Input: part model. Units: mm. Frame: model coordinates. A direction names the side the tool comes from. Coordinates: 2 decimals unless noted, no trailing zeros. Use one line per item in the form item = value.
Autodesk Inventor part; units mm, degrees
ref_plane "YZ Plane" through (0, 0, 0) normal (1, 0, 0) x (0, 1, 0)
ref_plane "XZ Plane" through (0, 0, 0) normal (0, 1, 0) x (-1, 0, 0)
ref_plane "XY Plane" through (0, 0, 0) normal (0, 0, 1) x (1, 0, 0)
ref_plane "Work Plane1" through (-701.2547, 0, 0) normal (0, 0, 1) x (1, 0, 0)
sketch "Sketch1" plane through (-701.2547, 0, 0) normal (0, 0, 1) x (1, 0, 0)
  line L0 (557.3903, 26) -> (429.8698, 26)
  arc A0 (429.8698, 26) -> (429.8698, 4) centre (429.8698, 15) ccw
  line L1 (429.8698, 4) -> (557.3903, 4)
  arc A1 (557.3903, 4) -> (557.3903, 26) centre (557.3903, 15) ccw
  line L2 (701.2547, 0) -> (1.2547, 0)
  line L3 (1.2547, 0) -> (1.2547, 30)
  line L4 (1.2547, 30) -> (701.2547, 30)
  line L5 (701.2547, 30) -> (701.2547, 0)
  line L6 (1.2547, 0) -> (701.2547, 0)
  line L7 (701.2547, 0) -> (701.2547, -50)
  line L8 (701.2547, -50) -> (1.2547, -50)
  line L9 (1.2547, -50) -> (1.2547, 0)
  line L10 (1.2547, -50) -> (31.2547, -700) construction
  line L11 (31.2547, -700) -> (351.2547, -850) construction
  line L12 (351.2547, -850) -> (671.2547, -700) construction
  line L13 (671.2547, -700) -> (701.2547, -50) construction
  spline S0 degree 4 poles (1.2547, -50) (31.2547, -700) (351.2547, -850) (671.2547, -700) (701.2547, -50) knots 1 1 1 1 1 2 2 2 2 2
  dimension "d0" = 50
  dimension "d1" = 850
  dimension "d2" = 700
  dimension "d3" = 30
  dimension "d4" = 30
  dimension "d5" = 350
  dimension "d6" = 350
extrude "Extrusion1" add sketch "Sketch1" along normal blind 25 contours L7 L8 L9 L2 | S0 L8
ref_plane "Work Plane2" through (-700, 0, 1930) normal (-1, 0, 0) x (0, 1, 0)
sketch "Sketch3" plane through (-700, -50, 0) normal (-1, 0, 0) x (0, 0, 1)
  circle A0 centre (37.5, 36) radius 12.5
  line L0 (0, 50) -> (25, 50)
  line L1 (25, 50) -> (25, 0)
  circle A1 centre (37.5, 36) radius 10
  arc A2 (40.5, 23.8653) -> (25, 13.8653) centre (45.3472, -0.6603) ccw
  line L2 (37.5, 48.5) -> (25, 48.5)
  point P0 (12.5, 50)
  point P1 (39.7301, 23.7006)
  point P2 (25, 36)
  point P3 (25, 41.0707)
  dimension "d11" = 12.5
  dimension "d12" = 2.5
  dimension "d13" = 20
  dimension "d14" = 10
  dimension "d15" = 3
  dimension "d16" = 25
  dimension "d17" = 14
  dimension "d18" = 12.5
extrude "Extrusion2" add sketch "Sketch3" against normal blind 30
fillet "Fillet1" radius 25 1 edges at (-350, 0, 0)
pattern_linear "Rectangular Pattern1" count 12 spacing 60 along (1, 0, 0) of "Extrusion2"
properties part number "back-flaps-3"
Q1. Set-up query: faces 4 (the flat face through (-430, -20, 29)), 5 (the cylindrical face through (-25.21, -11, 47.04)). Return all of +Z, -Z, +X, -X, +Y, -Y with unobstructed straight access to the full face (end or side cutting, diameter ignored); none if empty.
Check values:
face_4 = +Z, +Y, -Y
face_5 = +X, -X
Q2. First-contact query: P1, Ø20, axis at y = -25.5, z = 35.5, coming from the +X side; P2, Ø10, axis at y = -161.5, z = 26.5, coming from the -X side; P3, Ø1.5, axis at x = -276, y = -490, coming from the +Z side; P4, Ø18, axis at y = -14, z = 37.5, coming from the -X side. Flat tips, straight axial feed; report the tip coordinate or a pass-through.
Check values:
P1 = -10
P2 = -691.67
P3 = 25
P4 = through
Q3. Cut plane A-A, the plane y = -14. Give the number of separate pieces and of enclosed holes in the cut face, then the cut area to 3 significant figures.
Check values:
separate_pieces = 13
enclosed_holes = 0
area = 17,500 mm²
Q4. Ray query, line 1 along Z through (x, y) = (-105, -331.5); line 2 along Y through (x, z) = (-142, 41); line 3 along Y through (x, z) = (-571, 37). Return the intervals inside material, ascending. Write a range as [from, to].
Check values:
line_1 = [0, 25]
line_2 = [-26, -23.37], [-4.63, -2]
line_3 = [-27.09, -23.99], [-4.01, -1.5]
Q5. Pull-direction query (X, two-part tool) for faces 1 (the flat face through (-10, -20, 29)), 2 (the cylindrical face through (-385.21, -13.14, 49.97)), 3 (the flat face through (-580, -20, 29)); classes: pulls with the +X half, pulls with the -X half, needs draft (parallel to the pull), parting line crosses it, or undercut.
Check values:
face_1 = pulls with the +X half
face_2 = needs draft
face_3 = undercut
